Check sheet for the modelled part. Datum: model origin and axes. Units: mm. A direction names the side the tool comes from. Coordinates: 2 decimals unless noted, no trailing zeros. Write each loop counter-clockwise with the first axis right and the second up, starting at its lowest first coordinate (ties: lowest second). Pieces come first, ordered by that corner, then holes. Notation, with made-up numbers: (72.5, -17.75) - (91.5, -17.75) arc R29 ccw to (91.5, 21.25) - close; hole circle Ø11 at (88, 3). An arc over 180 degrees is marked (long way). Use one line per item in the form item = value. Start each with the question number.
1. Scan lines: line 1 along Y through (x, z) = (17, -13.5); line 2 along Z through (x, y) = (64, 2.75). Record each from-to range of solid material in increasing order.
2. Cross-section at B-B on x = 32.5. Record the boundary of the cut face in (y, z), then the cut area to 3 significant figures.
3. Draft check along Y on faces 3 (the face through (73.54, 9.79, -10.57)), 4 (the face through (29, 11.316, -8)), 5 (the face through (41.039, -8.856, 1.479)). Enter one of: +Y half, -Y half, draft (parallel to the pull), parting line (faces both ways), or undercut.
4. Cross-section at A-A on z = -10. Record the boundary of the cut face in (x, y).
5. Go/stop test with flat-tipped pins: pin 1 Ø2 at (x, z) = (56, -2.5) entering from -Y; pin 2 Ø8 at (x, y) = (20, -12) entering from -Z. Record where each tip stops, or that it passes through.
6. Tool access check on faces 1 (the face through (74.904, 2, 1)), 2 (the face through (27, -5, 0)). Record the directions out of +Z, -Z, +X, -X, +Y, -Y that give a thin tool (end or side, any length) a straight path to the whole face; none if there is none.
7. Cross-section at D-D on y = 5.5. Record the boundary of the cut face in (x, z).
8. Cross-section at C-C on z = -17.75. Record the boundary of the cut face in (x, y).
```python
from build123d import *

# Parameters (mm, degrees)
SKETCH_1_W          = 93.5
SKETCH_1_H          = 30
EXTRUDE_1_DEPTH     = 3
SKETCH_2_W          = 93.5
SKETCH_2_H          = 3
EXTRUDE_2_DEPTH     = 20
SKETCH_3_R          = 1.5
CUT_EXTRUDE_1_DEPTH = 20
SKETCH_4_R          = 1.5
CUT_EXTRUDE_2_DEPTH = 20


with BuildPart() as part:
    # 草图1 → 凸台-拉伸1 (new body)
    with BuildSketch(Plane.XY):
        with Locations((28.153508772, -3.684210526)):
            Rectangle(SKETCH_1_W, SKETCH_1_H)
    extrude(amount=EXTRUDE_1_DEPTH)

    # 草图2 → 凸台-拉伸2 (add)
    with BuildSketch(Plane(origin=(0, 0, 0), x_dir=(-1, 0, 0), z_dir=(0, 0, -1))):
        with Locations((-28.153508772, 9.815789474)):
            Rectangle(SKETCH_2_W, SKETCH_2_H)
    extrude(amount=EXTRUDE_2_DEPTH)

    # 草图3 → 切除-拉伸1 (cut)
    with BuildSketch(Plane.XZ.offset(-8.315789474)):
        with Locations((-15.846491228, -10)):
            Circle(SKETCH_3_R)
        with Locations((72.153508772, -10)):
            Circle(SKETCH_3_R)
    extrude(amount=-CUT_EXTRUDE_1_DEPTH, mode=Mode.SUBTRACT)

    # 草图4 → 切除-拉伸2 (cut)
    with BuildSketch(Plane(origin=(0, 0, 0), x_dir=(-1, 0, 0), z_dir=(0, 0, -1))):
        with Locations((-40.843508772, -10.343453639)):
            Circle(SKETCH_4_R)
        with Locations((-15.463508772, -10.343453639)):
            Circle(SKETCH_4_R)
    extrude(amount=-CUT_EXTRUDE_2_DEPTH, mode=Mode.SUBTRACT)


solid = part.part
```
Final values:
q1.line_1 = 8.32 to 11.32
q1.line_2 = 0 to 3
q2.outline = (-18.68, 0) - (8.32, 0) - (8.32, -20) - (11.32, -20) - (11.32, 3) - (-18.68, 3) - close
q2.area = 150 mm²
q3.face_3 = draft
q3.face_4 = +Y half
q3.face_5 = undercut
q4.outline = (-18.6, 8.32) - (-17.35, 8.32) - (-17.35, 11.32) - (-18.6, 11.32) - close; (-14.35, 8.32) - (70.65, 8.32) - (70.65, 11.32) - (-14.35, 11.32) - close; (73.65, 8.32) - (74.9, 8.32) - (74.9, 11.32) - (73.65, 11.32) - close
q5.pin_1 = 8.32
q5.pin_2 = 0
q6.face_1 = +Z, -Z, +X, +Y, -Y
q6.face_2 = -Z, +X, -X, -Y
q7.outline = (-18.6, 0) - (74.9, 0) - (74.9, 3) - (-18.6, 3) - close
q8.outline = (-18.6, 8.32) - (74.9, 8.32) - (74.9, 11.32) - (-18.6, 11.32) - close
